The model under review builds one solid part; all positions refer to its coordinate system, in mm. Face numbers are marked on the shaded views. A direction names the side the tool comes from. Round coordinates to 2 decimals unless told otherwise and drop trailing zeros. Write each loop counter-clockwise with the first axis right and the second up, starting at its lowest first coordinate (ties: lowest second). Pieces come first, ordered by that corner, then holes. Notation, with made-up numbers: (29, 56) - (37, 56) arc R14 cw to (37, 70) - close; hole circle Ø5 at (76, 8). An arc over 180 degrees is marked (long way). One line per question, with ' | ' between items. Start each with the question number.
```python
from build123d import *

# Parameters (mm, degrees)
ESBO_O1_W                      = 34
ESBO_O1_H                      = 30
RESSALTO_EXTRUS_O1_DEPTH       = 22
CORTE_EXTRUS_O1_DEPTH          = 31
CORTE_EXTRUS_O2_DEPTH          = 31
CORTE_EXTRUS_O3_DEPTH          = 31
CORTE_EXTRUS_O4_DEPTH          = 31
CORTE_EXTRUS_O5_DEPTH          = 31
FURO_DE_DI_METRO_4_0_4_1_D     = 4
FURO_DE_DI_METRO_4_0_4_1_DEPTH = 18
FURO_DE_DI_METRO_4_0_4_2_D     = 4
FURO_DE_DI_METRO_4_0_4_2_DEPTH = 22
CHANFRO1_SIZE                  = 1.5
CHANFRO2_SIZE                  = 0.500000009


with BuildPart() as part:
    # Esboço1 → Ressalto-extrusão1 (new body)
    with BuildSketch(Plane(origin=(0, 13.318571188, 0), x_dir=(1, 0, 0), z_dir=(0, 1, 0))):
        with Locations((0.093581821, -15)):
            Rectangle(ESBO_O1_W, ESBO_O1_H)
    extrude(amount=-RESSALTO_EXTRUS_O1_DEPTH)

    # Esboço2 → Corte-extrusão1 (cut, through all)
    with BuildSketch(Plane(origin=(0, 0, 0), x_dir=(-1, 0, 0), z_dir=(0, 0, -1))):
        Polygon((-17.093581821, -2.181428812), (-16.093581821, -1.181428812), (-16.093581821, 13.318571188), (-17.093581821, 13.318571188), align=None)
    extrude(amount=-CORTE_EXTRUS_O1_DEPTH, mode=Mode.SUBTRACT)

    # Esboço3 → Corte-extrusão2 (cut, through all)
    with BuildSketch(Plane(origin=(0, 0, 0), x_dir=(-1, 0, 0), z_dir=(0, 0, -1))):
        Polygon((-16.093581821, 13.318571188), (-16.093581821, 9.318571188), (-8.093581821, 9.318571188), (-4.093581821, 13.318571188), align=None)
    extrude(amount=-CORTE_EXTRUS_O2_DEPTH, mode=Mode.SUBTRACT)

    # Esboço4 → Corte-extrusão3 (cut, through all)
    with BuildSketch(Plane(origin=(0, 0, 0), x_dir=(-1, 0, 0), z_dir=(0, 0, -1))):
        Polygon((16.906418179, 13.318571188), (3.906418179, 13.318571188), (7.906418179, 9.318571188), (16.906418179, 9.318571188), align=None)
    extrude(amount=-CORTE_EXTRUS_O3_DEPTH, mode=Mode.SUBTRACT)

    # Esboço5 → Corte-extrusão4 (cut, through all)
    with BuildSketch(Plane(origin=(0, 0, 0), x_dir=(-1, 0, 0), z_dir=(0, 0, -1))):
        Polygon((15.906418179, 9.318571188), (15.906418179, -1.181428812), (16.906418179, -2.181428812), (16.906418179, 9.318571188), align=None)
    extrude(amount=-CORTE_EXTRUS_O4_DEPTH, mode=Mode.SUBTRACT)

    # Esboço6 → Corte-extrusão5 (cut, through all)
    with BuildSketch(Plane(origin=(0, 0, 0), x_dir=(-1, 0, 0), z_dir=(0, 0, -1))):
        Polygon((-4.593581821, -8.681428812), (4.406418179, -8.681428812), (3.906418179, -8.181428812), (-4.093581821, -8.181428812), align=None)
    extrude(amount=-CORTE_EXTRUS_O5_DEPTH, mode=Mode.SUBTRACT)

    # Esboço7 → Corte-Revolução1 (revolve, cut)
    with BuildSketch(Plane.XZ.offset(-2.318571188)):
        Polygon((7.593581821, 30), (0.093581821, 30), (0.093581821, 0), (7.593581821, 0), (7.593581821, 1), (4.118581821, 1), (4.118581821, 29), (7.593581821, 29), align=None)
    revolve(axis=Axis((0.093581821, 2.318571188, 30), (0, 0, -1)), mode=Mode.SUBTRACT)

    # Furo de diâmetro Ø4.0 (4)1
    with Locations(Plane(origin=(0, 9.318571188, 0), x_dir=(1, 0, 0), z_dir=(0, 1, 0))):
        with Locations((12.093581821, -24)):
            Hole(FURO_DE_DI_METRO_4_0_4_1_D / 2, depth=FURO_DE_DI_METRO_4_0_4_1_DEPTH)

    # Furo de diâmetro Ø4.0 (4)2
    with Locations(Plane(origin=(0, -8.681428812, 0), x_dir=(-1, 0, 0), z_dir=(0, -1, 0))):
        with Locations((11.906418179, -6), (11.906418179, -24), (-12.093581821, -6)):
            Hole(FURO_DE_DI_METRO_4_0_4_2_D / 2, depth=FURO_DE_DI_METRO_4_0_4_2_DEPTH)

    # Chanfro1
    chanfro1_edges = [part.edges().sort_by_distance(p)[0] for p in [
        (17.093581821, -8.681428812, 15),
        (-16.906418179, -8.681428812, 15),
    ]]
    chamfer(chanfro1_edges, length=CHANFRO1_SIZE)

    # Chanfro2
    chanfro2_edges = [part.edges().sort_by_distance(p)[0] for p in [
        (10.093581821, 9.318571188, 6),
        (10.093581821, -8.681428812, 6),
        (-13.906418179, 9.318571188, 24),
        (-13.906418179, -8.681428812, 24),
        (-13.906418179, 9.318571188, 6),
        (-13.906418179, -8.681428812, 6),
        (17.093581821, -4.681428812, 30),
        (17.093581821, -4.681428812, 0),
        (-16.906418179, -4.681428812, 0),
        (-16.156418179, -7.931428812, 0),
        (16.343581821, -7.931428812, 0),
        (-16.906418179, -4.681428812, 30),
        (-16.156418179, -7.931428812, 30),
        (16.343581821, -7.931428812, 30),
        (16.093581821, 4.068571188, 30),
        (16.593581821, -1.681428812, 30),
        (16.593581821, -1.681428812, 0),
        (16.093581821, 4.068571188, 0),
        (0.093581821, 13.318571188, 0),
        (6.093581821, 11.318571188, 30),
        (12.093581821, 9.318571188, 30),
        (16.093581821, 9.318571188, 15),
        (12.093581821, 9.318571188, 0),
        (6.093581821, 11.318571188, 0),
        (0.093581821, 13.318571188, 30),
        (-11.906418179, 9.318571188, 30),
        (-5.906418179, 11.318571188, 30),
        (-5.906418179, 11.318571188, 0),
        (-11.906418179, 9.318571188, 0),
        (-15.906418179, 9.318571188, 15),
        (-16.406418179, -1.681428812, 30),
        (-15.906418179, 4.068571188, 30),
        (-15.906418179, 4.068571188, 0),
        (-16.406418179, -1.681428812, 0),
        (14.093581821, 9.318571188, 24),
        (14.093581821, -8.681428812, 24),
    ]]
    chamfer(chanfro2_edges, length=CHANFRO2_SIZE)


solid = part.part
```
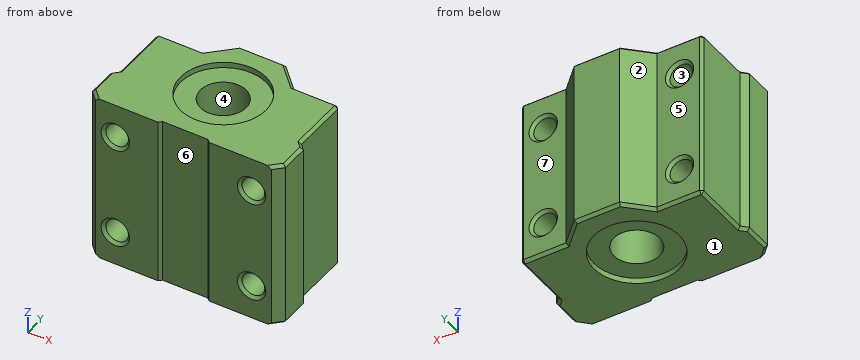
1. Add section B-B, the plane z = 9.5. Write out the cut boundary in (x, y) (3 decimals), then the cut area to 3 significant figures.
2. Add section C-C, the plane x = -8.5. Write out the cut boundary in (y, z).
3. Machinability: for the marked faces 5, 6 and 7, which of the approach directions +Z, -Z, +X, -X, +Y, -Y give a long, thin tool a straight path to every point of the face, cutting with its end or side? Answer none if there is none.
4. Add section A-A, the plane y = -0.25. Write out the cut boundary in (x, z).
5. Add section D-D, the plane z = 24. State how many separate pieces and enclosed holes the cut face has, then the cut area to 3 significant figures.
6. Wall thickness on line 1 along X through (y, z) = (-4.5, 24); line 2 along X through (y, z) = (-5, 5.5); line 3 along X through (y, z) = (0.75, 24): over which ranges is each line inside the solid? List them lowest first. Write a range as [from, to].
7. The part is to be moulded in two halves that separate along X. For the marked faces 1, 2, 3 and 4, say which applies: pulls with the +X half, pulls with the -X half, needs draft (parallel to the pull), parting line crosses it, or undercut.
8. Clearance check with flat-ended pins moving along their axes: P1, Ø6, axis at y = 3, z = 8, coming from the +X side; P2, Ø8, axis at x = 10, z = 20.5, coming from the +Y side; P3, Ø8, axis at x = 12, z = 21.5, coming from the +Y side. State where each tip first meets the part, or that it passes through.
Geometry check:
1) outline: (-16.906, -7.181) - (-15.406, -8.681) - (-4.406, -8.681) - (-3.906, -8.181) - (4.094, -8.181) - (4.594, -8.681) - (15.594, -8.681) - (17.094, -7.181) - (17.094, -2.181) - (16.094, -1.181) - (16.094, 8.819) - (15.594, 9.319) - (8.094, 9.319) - (4.094, 13.319) - (-3.906, 13.319) - (-7.906, 9.319) - (-15.406, 9.319) - (-15.906, 8.819) - (-15.906, -1.181) - (-16.906, -2.181) - close; hole circle Ø8.05 at (0.094, 2.319) | area: 580 mm2
2) outline: (-8.68, 0) - (8.82, 0) - (9.32, 0.5) - (9.32, 29.5) - (8.82, 30) - (-8.68, 30) - close
3) face 5: +Z, -Z, -X, +Y | face 6: +Z, -Z, -Y | face 7: +Z, -Z, +X, +Y
4) outline: (-15.91, 0.5) - (-15.41, 0) - (-6.95, 0) - (-6.95, 1) - (-3.01, 1) - (-3.01, 29) - (-6.95, 29) - (-6.95, 30) - (-15.41, 30) - (-15.91, 29.5) - close; (3.19, 1) - (7.14, 1) - (7.14, 0) - (15.59, 0) - (16.09, 0.5) - (16.09, 29.5) - (15.59, 30) - (7.14, 30) - (7.14, 29) - (3.19, 29) - close; hole circle Ø4 at (-11.91, 6); hole circle Ø4 at (-11.91, 24); hole circle Ø4 at (12.09, 6); hole circle Ø4 at (12.09, 24)
5) separate pieces: 3 | enclosed holes: 1 | area: 435 mm2
6) line 1: x = [-16.91, -13.91], [-9.91, 10.09], [14.09, 17.09] | line 2: x = [-16.91, -13.84], [-9.97, 10.16], [14.03, 17.09] | line 3: x = [-15.91, -13.91], [-9.91, -3.61], [3.8, 10.09], [14.09, 16.09]
7) face 1: needs draft | face 2: pulls with the -X half | face 3: undercut | face 4: undercut
8) P1: stops at x = 16.09 | P2: stops at y = 11.41 | P3: stops at y = 9.41
